Input: dimensioned drawing with shaded views. Units: mm. Origin: part minimum x, y, z. Give positions to 0.01 mm unless a question says otherwise; leave off trailing zeros. Loops run counter-clockwise (first coordinate to the right, second up) from the corner with the lowest first, then second, coordinate; pieces in that order, holes last.
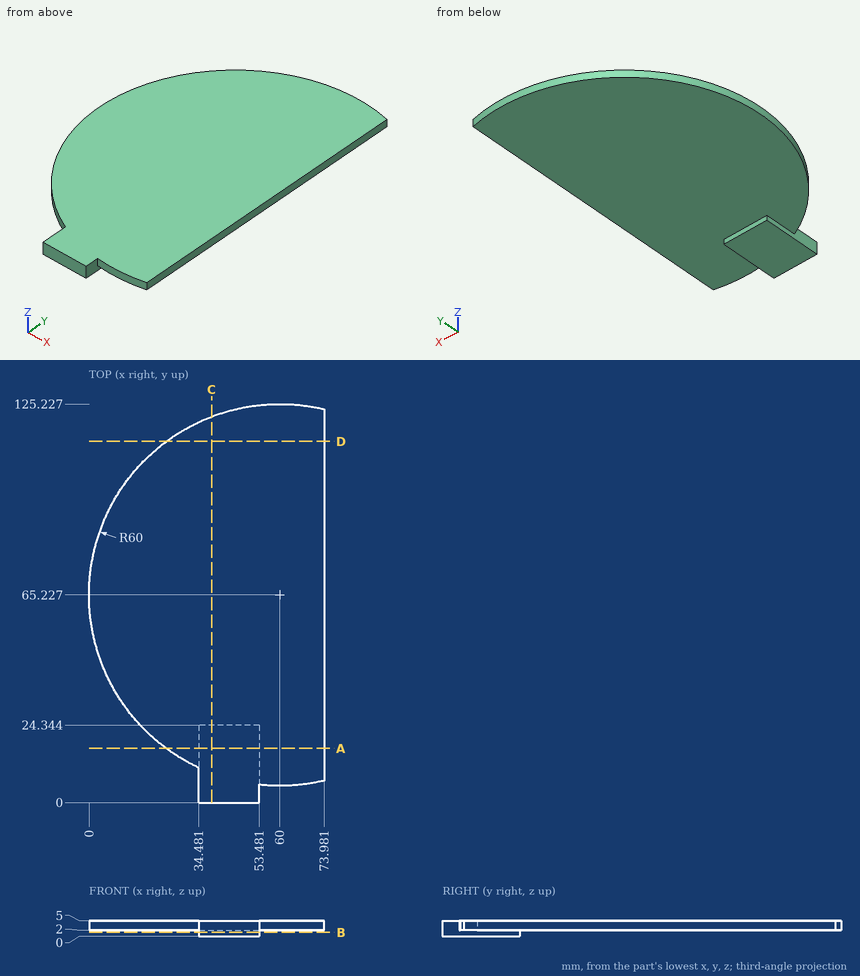
Item 1: Section query D-D on y = 113.5. Return loops of the section in (x, z).
Values follow:
outline: (24.37, 2) - (73.98, 2) - (73.98, 5) - (24.37, 5) - close
Item 2: Section query A-A on y = 17. Return loops of the section in (x, z) (1 decimal), plus the area to 3 significant figures.
Values follow:
outline: (24.3, 2) - (34.5, 2) - (34.5, 0) - (53.5, 0) - (53.5, 2) - (74, 2) - (74, 5) - (24.3, 5) - close
area: 187 mm2
Item 3: Ray query, probe 1 along Z at (x, y) = (58.5, 17); probe 2 along Y at (x, z) = (50.5, 1.25); probe 3 along X at (y, z) = (107.5, 4.55). Return the intervals inside material, ascending.
Values follow:
probe 1: z = 2 to 5
probe 2: y = 0 to 24.34
probe 3: x = 17.42 to 73.98
Item 4: Section query C-C on x = 38.5. Return loops of the section in (y, z).
Values follow:
outline: (0, 0) - (24.34, 0) - (24.34, 2) - (121.24, 2) - (121.24, 5) - (0, 5) - close
Item 5: Pin query (flat end, axial travel): pin 1 (4 mm diameter, centred on x = 44, y = 70, fed in from -Z); pin 2 (2 mm diameter, centred on x = 41.5, z = 1.5, fed in from +Y). Return the tip coordinate at first contact, or that it passes through.
Values follow:
pin 1: stops at z = 2
pin 2: stops at y = 122.58
Item 6: Section query B-B on z = 1.25. Return loops of the section in (x, y).
Values follow:
outline: (34.48, 0) - (53.48, 0) - (53.48, 24.34) - (34.48, 24.34) - close
